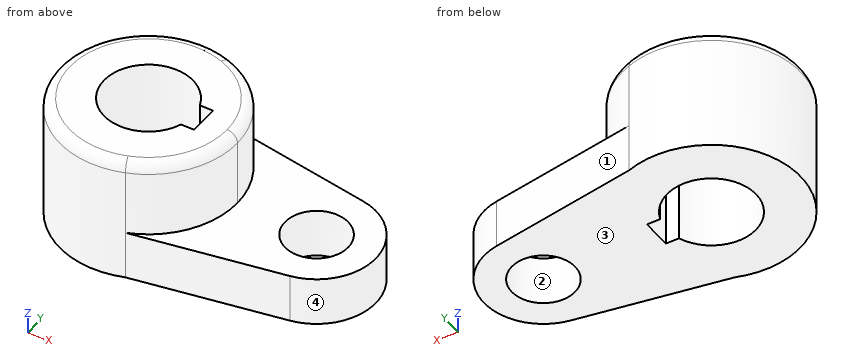
from build123d import *

# Parameters (mm, degrees)
F0_R     = 26.8981643916
F1_DEPTH = 40.2336
F0_R_2   = 10.16
F2_DEPTH = 15.7734
F3_R     = 3.302


with BuildPart() as f1:
    # F0 (on Top) → F1 (new body)
    with BuildSketch(Plane.XY):
        with BuildLine():
            ThreePointArc((9.5121844836, -26.9452959039), (23.3274655355, -16.5033322905), (28.575, 0))
            ThreePointArc((28.575, 0), (23.3274655355, 16.5033322905), (9.5121844836, 26.9452959039))
            ThreePointArc((9.5121844836, 26.9452959039), (-28.575, 0), (9.5121844836, -26.9452959039))
        make_face()
        Circle(F0_R, mode=Mode.SUBTRACT)
        Circle(F0_R)
        with BuildLine():
            ThreePointArc((13.4477648793, -4.826), (-14.2875, 0), (13.4477648793, 4.826))
            Line((13.4477648793, 4.826), (17.6895648793, 4.826))
            Line((17.6895648793, 4.826), (17.6895648793, -4.826))
            Line((17.6895648793, -4.826), (13.4477648793, -4.826))
        make_face(mode=Mode.SUBTRACT)
    extrude(amount=F1_DEPTH)

    # F0 (on Top) → F2 (join)
    with BuildSketch(Plane.XY):
        with BuildLine():
            ThreePointArc((9.5121844836, 26.9452959039), (23.3274655355, 16.5033322905), (28.575, 0))
            ThreePointArc((28.575, 0), (23.3274655355, -16.5033322905), (9.5121844836, -26.9452959039))
            Line((9.5121844836, -26.9452959039), (57.1919272622, -18.7764181619))
            ThreePointArc((57.1919272622, -18.7764181619), (73.025, 0), (57.1919272622, 18.7764181619))
            Line((57.1919272622, 18.7764181619), (9.5121844836, 26.9452959039))
        make_face()
        with Locations((53.975, 0)):
            Circle(F0_R_2, mode=Mode.SUBTRACT)
    extrude(amount=F2_DEPTH)

    # F3
    f3_edges = [f1.edges().sort_by_distance(p)[0] for p in [
        (-9.512184, 26.945296, 40.2336),
    ]]
    fillet(f3_edges, radius=F3_R)


solid = f1.part
Read the model definition and answer for the solid it produces. Units are mm, in the model's axes. Face numbers are marked on the shaded views. Give positions to 0.01 mm unless a question says otherwise; leave off trailing zeros. Write each loop counter-clockwise with the first axis right and the second up, starting at its lowest first coordinate (ties: lowest second). Pieces come first, ordered by that corner, then holes. Notation, with made-up numbers: (20, -38.5) - (63, -38.5) arc R33 ccw to (63, -7.5) - close; hole circle Ø7 at (39.25, 49). An arc over 180 degrees is marked (long way). Use CSV: the item, a comma, the result in double quotes. Start each with the question number.
Item 1: The mould has two halves that part along Y. Classify the marked faces 1, 2, 3 and 4: pulls with the +Y half, pulls with the -Y half, needs draft (parallel to the pull), parting line crosses it, or undercut.
Item 2: Flat-ended cylindrical pins translate along their axes: P1, Ø1.5, axis at y = -9.5, z = 18.5, coming from the -X side; P2, Ø10, axis at y = 14.5, z = 34, coming from the +X side; P3, Ø2, axis at x = 22.5, z = 26, coming from the -Y side; P4, Ø2, axis at x = 13.5, y = -5, coming from the -Z side. Find the tip coordinate at first contact, or state that the pin passes through.
Item 3: Consider line 1 (Y direction, x = 0, z = 16) (1 decimal); line 2 (X direction, y = 0, z = 29) (1 decimal); line 3 (Y direction, x = 55, z = 6). Determine where each line is inside the solid, lowest interval first.
Item 4: The part is cut by section A-A, the plane z = 13.5. Count the separate pieces of the cut face and the enclosed holes in it, and give its area (3 significant figures).
Item 5: The part is cut by section D-D, the plane x = 33.5. Give the vertices of the cut face in (y, z), and give its area (3 significant figures).
Taken from the geometry:
1,face 1,"pulls with the +Y half"
1,face 2,"undercut"
1,face 3,"needs draft"
1,face 4,"parting line crosses it"
2,P1,"x = -27.2"
2,P2,"x = 26.95"
2,P3,"y = -18.82"
2,P4,"z = 0"
3,line 1,"-28.6 to -14.3, 14.3 to 28.6"
3,line 2,"-28.6 to -14.3, 17.7 to 28.6"
3,line 3,"-19.15 to -10.11, 10.11 to 19.15"
4,separate pieces,"1"
4,enclosed holes,"2"
4,area,"3,440 mm2"
5,outline,"(-22.84, 0) - (22.84, 0) - (22.84, 15.77) - (-22.84, 15.77) - close"
5,area,"720 mm2"
